For this review, take the finished solid that the model builds, in its own axes (mm). A direction names the side the tool comes from. Give positions to 0.01 mm unless a question says otherwise; leave off trailing zeros. Order: outer loops, then holes, each group sorted by start corner. A loop starts at its lowest first (then second) coordinate and runs counter-clockwise, first axis right, second up. Notation, with made-up numbers: (46.25, 24) - (59.25, 24) arc R17 ccw to (59.25, 47) - close; hole circle Ø8 at (19, 79). An arc over 180 degrees is marked (long way). Use a Markdown table: item, result. Add a question column.
1) Clearance check with flat-ended pins moving along their axes: P1, Ø2, axis at x = 2.5, z = -9, coming from the +Y side; P2, Ø1, axis at x = 11, z = 3, coming from the -Y side; P3, Ø12.5, axis at x = 1.5, z = 2.5, coming from the +Y side. State where each tip first meets the part, or that it passes through.
2) We need section C-C on y = 5.5. Write out the cut boundary in (x, z).
3) We need section D-D on x = 0. Write out the cut boundary in (y, z).
4) Machinability: for faces 5 (the face through (0, 31.5, -7.5)), 6 (the face through (0, 15, 10.5)), 7 (the face through (0, 31.7, -6.5)), 8 (the face through (0, 15, 12.5)), which of the approach directions +Z, -Z, +X, -X, +Y, -Y give a long, thin tool a straight path to every point of the face, cutting with its end or side? Answer none if there is none.
5) We need section A-A on z = 7.5. Write out the cut boundary in (x, y), then the cut area to 3 significant figures.
6) Wall thickness on L1, parallel to X at y = 3.5, z = 5.25; L2, parallel to Z at x = 7.5, y = 6; L3, parallel to Y at x = -8.5, z = 2.75: over which ranges is each line inside the solid? List them lowest first.
7) We need section B-B on x = -3.25. Write out the cut boundary in (y, z).
8) Mouldability with a two-part tool opening along X and no side actions: class faces 1 (the face through (7.75, 15, 5)), 2 (the face through (14.699, 15.21, -12.215)), 3 (the face through (-7.75, 15, 5)), 4 (the face through (0, 31.7, -8.5)) as released by +X, released by -X, zero draft, split by the parting line, or undercut.
```python
from build123d import *

# Parameters (mm, degrees)
SKETCH1_W           = 30
SKETCH1_H           = 25
BOSS_EXTRUDE1_DEPTH = 30
SKETCH2_W           = 15.5
SKETCH2_H           = 12
CUT_EXTRUDE1_DEPTH  = 30
FILLET1_R           = 1
BOSS_EXTRUDE2_DEPTH = 1


with BuildPart() as part:
    # Sketch1 → Boss-Extrude1 (new body)
    with BuildSketch(Plane(origin=(0, 0, 0), x_dir=(1, 0, 0), z_dir=(0, 1, 0))):
        Rectangle(SKETCH1_W, SKETCH1_H)
    extrude(amount=BOSS_EXTRUDE1_DEPTH)

    # Sketch2 → Cut-Extrude1 (cut)
    with BuildSketch(Plane(origin=(0, 30, 0), x_dir=(1, 0, 0), z_dir=(0, 1, 0))):
        with Locations((0, -4.5)):
            Rectangle(SKETCH2_W, SKETCH2_H)
    extrude(amount=-CUT_EXTRUDE1_DEPTH, mode=Mode.SUBTRACT)

    # Fillet1
    fillet1_edges = [part.edges().sort_by_distance(p)[0] for p in [
        (15, 15, 12.5),
        (-15, 15, 12.5),
        (-15, 15, -12.5),
        (15, 15, -12.5),
    ]]
    fillet(fillet1_edges, radius=FILLET1_R)

    # Sketch3 → Boss-Extrude2 (add, symmetric)
    with BuildSketch(Plane(origin=(0, 0, -7.5), x_dir=(-1, 0, 0), z_dir=(0, 0, -1))):
        with BuildLine():
            ThreePointArc((2, 30), (0, 32), (-2, 30))
            Line((-2, 30), (-1.5, 30))
            ThreePointArc((-1.5, 30), (0, 31.5), (1.5, 30))
            Line((1.5, 30), (2, 30))
        make_face()
    extrude(amount=BOSS_EXTRUDE2_DEPTH, both=True)


solid = part.part
```
Checked values:
| question | item | result |
|---|---|---|
| 1 | P1 | y = 31.15 |
| 1 | P2 | y = 0 |
| 1 | P3 | y = 30 |
| 2 | outline | (-15, -11.5) arc R1 ccw to (-14, -12.5) - (14, -12.5) arc R1 ccw to (15, -11.5) - (15, 11.5) arc R1 ccw to (14, 12.5) - (-14, 12.5) arc R1 ccw to (-15, 11.5) - close; hole (-7.75, -1.5) - (7.75, -1.5) - (7.75, 10.5) - (-7.75, 10.5) - close |
| 3 | outline | (0, -12.5) - (30, -12.5) - (30, -1.5) - (0, -1.5) - close; (0, 10.5) - (30, 10.5) - (30, 12.5) - (0, 12.5) - close; (31.5, -8.5) - (32, -8.5) - (32, -6.5) - (31.5, -6.5) - close |
| 4 | face 5 | +Z, -Z |
| 4 | face 6 | +Y, -Y |
| 4 | face 7 | +Z, +X, -X, +Y |
| 4 | face 8 | +Z, +X, -X, +Y, -Y |
| 5 | outline | (-15, 0) - (-7.75, 0) - (-7.75, 30) - (-15, 30) - close; (7.75, 0) - (15, 0) - (15, 30) - (7.75, 30) - close |
| 5 | area | 435 mm² |
| 6 | L1 | -15 to -7.75, 7.75 to 15 |
| 6 | L2 | -12.5 to -1.5, 10.5 to 12.5 |
| 6 | L3 | 0 to 30 |
| 7 | outline | (0, -12.5) - (30, -12.5) - (30, -1.5) - (0, -1.5) - close; (0, 10.5) - (30, 10.5) - (30, 12.5) - (0, 12.5) - close |
| 8 | face 1 | undercut |
| 8 | face 2 | released by +X |
| 8 | face 3 | undercut |
| 8 | face 4 | zero draft |
